Check sheet for the modelled part. Datum: model origin and axes. Units: mm. A direction names the side the tool comes from. Coordinates: 2 decimals unless noted, no trailing zeros. Order: outer loops, then holes, each group sorted by start corner. A loop starts at its lowest first (then second) coordinate and runs counter-clockwise, first axis right, second up.
1. Cross-section at B-B (x = 158.5). Enter the section's corners in (y, z), then the cut area to 3 significant figures.
2. Cross-section at A-A (x = -21). Enter the section's corners in (y, z), then the cut area to 3 significant figures.
3. Draft check along X on faces 4 (the cylindrical face through (6.515, -17.722, 56.275)), 5 (the conical face through (-16.42, 52.45, 27.28)), 6 (the flat face through (-1.541, -19.3, -8.7)), 7 (the flat face through (-29.541, -11, 41)). Enter one of: released by +X, released by -X, zero draft, split by the parting line, or undercut.
4. Gauge pin test, flat ends, axial feed: pin 1 Ø3 at (x, z) = (47, 7.5) entering from -Y; pin 2 Ø12 at (x, z) = (22.5, -36.5) entering from -Y; pin 3 Ø4 at (x, z) = (146.5, -2.5) entering from -Y. Record the tip position at first contact, or that the pin passes through.
5. Set-up check for faces 1 (the conical face through (113.887, -9.9, 31.436)), 2 (the cylindrical face through (-65.485, -17.722, 56.275)), 3 (the flat face through (-33.541, -41, -26)): record each of +Z, -Z, +X, -X, +Y, -Y from which the full face is reachable in a straight line by a thin tool's end or side.
6. Thickness scan on line 1 (Z direction, x = -2, y = -1); line 2 (Y direction, x = -67, z = 0); line 3 (Y direction, x = -55, z = 0). Record the ranges inside material, lowest first.
```python
from build123d import *


with BuildPart() as part:
    # Sketch1 → Revolve1 (revolve)
    with BuildSketch(Plane.XY, mode=Mode.PRIVATE) as revolve1_sk:
        with BuildLine():
            Line((-69.541046611, 59), (-61.541046611, 59))
            Line((-61.541046611, 59), (-59.541046611, 61))
            Line((-59.541046611, 61), (-44.541046611, 61))
            Line((-44.541046611, 61), (-42.541046611, 59))
            Line((-42.541046611, 59), (-16.541046611, 59))
            Line((-16.541046611, 59), (-14.541046611, 61))
            Line((-14.541046611, 61), (0.458953389, 61))
            Line((0.458953389, 61), (2.458953389, 59))
            Line((2.458953389, 59), (10.458953389, 59))
            Line((10.458953389, 59), (10.458953389, 36))
            Line((10.458953389, 36), (214.458953389, 30))
            Line((214.458953389, 30), (214.458953389, 21))
            Line((214.458953389, 21), (207.378173445, 21))
            ThreePointArc((207.378173445, 21), (206.378173445, 21.742044507), (205.378173445, 21))
            Line((205.378173445, 21), (190.378173445, 21))
            ThreePointArc((190.378173445, 21), (187.878173445, 22.035533906), (185.378173445, 21))
            Line((185.378173445, 21), (-1.541046611, 21))
            Line((-1.541046611, 21), (-1.541046611, 42))
            Line((-1.541046611, 42), (-29.541046611, 42))
            Line((-29.541046611, 42), (-29.541046611, 49.65729462))
            Line((-29.541046611, 49.65729462), (-33.541046611, 49.65729462))
            Line((-33.541046611, 49.65729462), (-33.541046611, 48))
            Line((-33.541046611, 48), (-79.541046611, 48))
            Line((-79.541046611, 48), (-69.541046611, 59))
        make_face()
    revolve(revolve1_sk.sketch.rotate(Axis((-185.161107322, 0, 0), (1, 0, 0)), 90), axis=Axis((-185.161107322, 0, 0), (1, 0, 0)))


solid = part.part
```
Data:
1. outline: circle Ø63.29 at (0, 0); hole circle Ø42 at (0, 0)
1. area: 1,760 mm2
2. outline: circle Ø118 at (0, 0); hole circle Ø84 at (0, 0)
2. area: 5,390 mm2
3. face 4: zero draft
3. face 5: undercut
3. face 6: released by -X
3. face 7: undercut
4. pin 1: stops at y = -34.41
4. pin 2: stops at y = -18.46
4. pin 3: stops at y = -32.02
5. face 1: +X
5. face 2: -X
5. face 3: none
6. line 1: z = -60.99 to -41.99, 41.99 to 60.99
6. line 2: y = -59 to -48, 48 to 59
6. line 3: y = -61 to -48, 48 to 61
